Answer from the drawing. Dimensions are ordinates in mm from the lowest x, y and z of the part. Round coordinates to 2 decimals unless told otherwise and drop trailing zeros. Order: outer loops, then holes, each group sorted by start corner. A loop starts at its lowest first (then second) coordinate and runs counter-clockwise, first axis right, second up. Notation, with made-up numbers: (-28.75, 77) -> (26.25, 77) arc R10 ccw to (26.25, 96) -> close; hole circle Ø4 at (79.5, 4.5). An arc over 180 degrees is marked (long way). Use a Markdown table: item, result. Add a question column.
Item 1: A cutting plane is placed at A-A, the plane y = 30. Determine the outline of the cut face in (x, z).
Item 2: A flat-ended cylindrical pin translates along its axis: P1, Ø2, axis at y = 10.5, z = 1, coming from the +X side. Find the tip coordinate at first contact, or state that the pin passes through.
Item 3: Find the intervals of material crossed by L1, parallel to Y at x = 50.5, z = 0.65 (1 decimal); L2, parallel to X at y = 50, z = 2.9; L3, parallel to X at y = 14, z = 4.2 (1 decimal), in increasing order. Write a range as [from, to].
Item 4: A cutting plane is placed at C-C, the plane y = 57.5. Determine the outline of the cut face in (x, z), plus the area to 3 significant figures.
Item 5: A cutting plane is placed at B-B, the plane x = 43. Determine the outline of the cut face in (y, z).
Item 6: For a pull along Y with two mould halves and no side action, classify the marked faces 1, 2 and 3 as +Y half, -Y half, draft (parallel to the pull), parting line (faces both ways), or undercut.
Item 7: A cutting plane is placed at D-D, the plane z = 0.75. Give the number of separate pieces and of enclosed holes in the cut face.
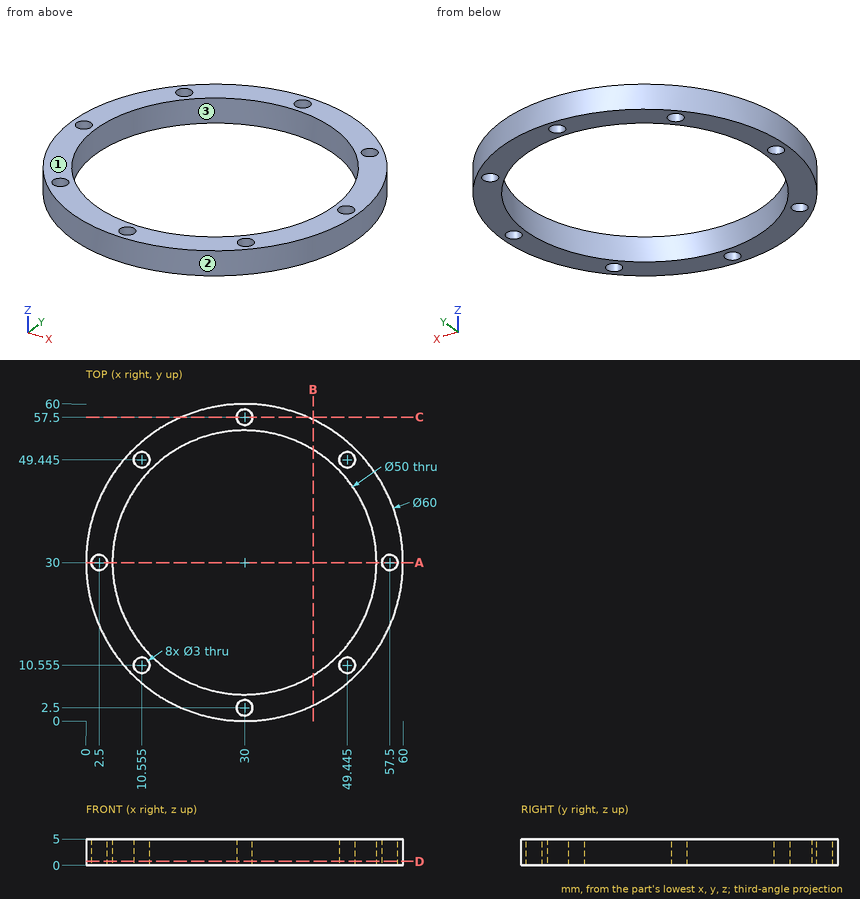
Reported:
| question | item | result |
|---|---|---|
| 1 | outline | (0, 0) -> (1, 0) -> (1, 5) -> (0, 5) -> close; (4, 0) -> (5, 0) -> (5, 5) -> (4, 5) -> close; (55, 0) -> (56, 0) -> (56, 5) -> (55, 5) -> close; (59, 0) -> (60, 0) -> (60, 5) -> (59, 5) -> close |
| 2 | P1 | x = 53.62 |
| 3 | L1 | [8.1, 9.5], [11.6, 15.7], [44.3, 48.4], [50.5, 51.9] |
| 3 | L2 | [7.64, 9.16], [11.95, 15], [45, 48.05], [50.84, 52.36] |
| 3 | L3 | [4.6, 10.8], [49.2, 55.4] |
| 4 | outline | (18.01, 0) -> (28.5, 0) -> (28.5, 5) -> (18.01, 5) -> close; (31.5, 0) -> (41.99, 0) -> (41.99, 5) -> (31.5, 5) -> close |
| 4 | area | 105 mm² |
| 5 | outline | (2.96, 0) -> (8.65, 0) -> (8.65, 5) -> (2.96, 5) -> close; (51.35, 0) -> (57.04, 0) -> (57.04, 5) -> (51.35, 5) -> close |
| 6 | face 1 | draft |
| 6 | face 2 | parting line |
| 6 | face 3 | undercut |
| 7 | separate pieces | 1 |
| 7 | enclosed holes | 9 |
